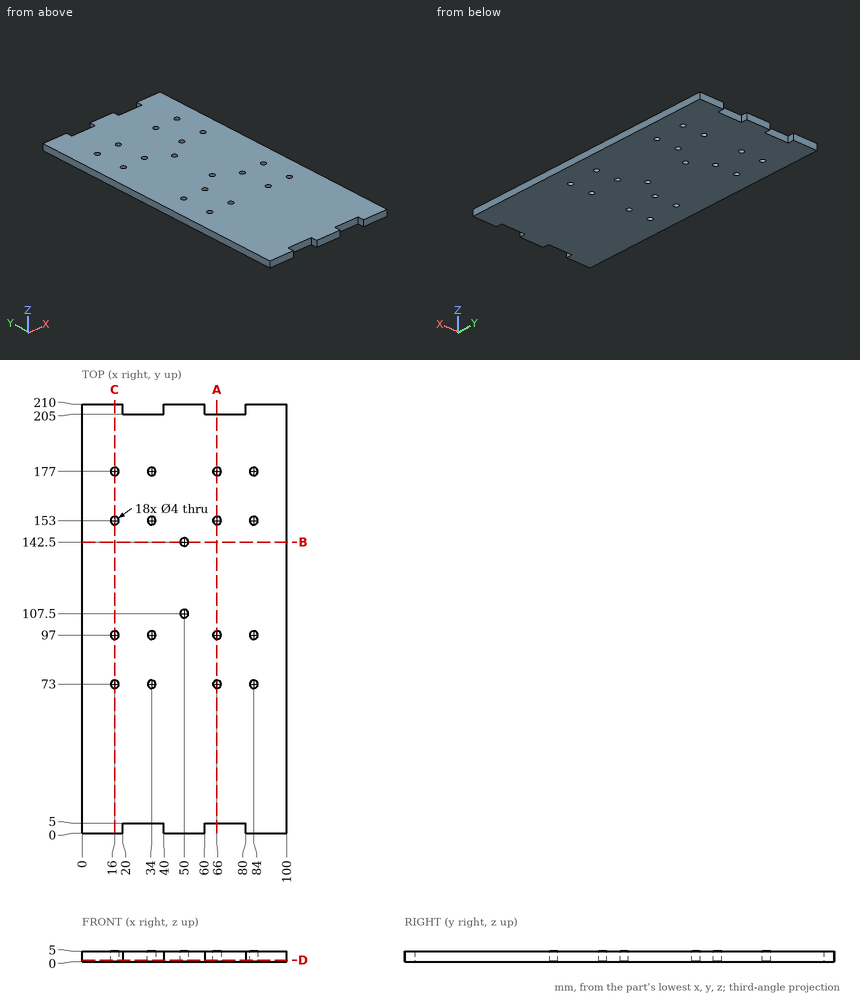
Verification items for this drawing (mm, ordinates from the low corner). Coordinates: 2 decimals unless noted, no trailing zeros. Write each loop counter-clockwise with the first axis right and the second up, starting at its lowest first coordinate (ties: lowest second). Pieces come first, ordered by that corner, then holes. Notation, with made-up numbers: M 63,18.5 L 70,18.5 A26 ccw 70,39.5 Z; hole C 81.5,10 d8. An arc over 180 degrees is marked long. Answer as CSV lines item,"result".
Q1. Cross-section at C-C (x = 16). Record the boundary of the cut face in (y, z).
Check result:
outline,"M 0,0 L 71,0 L 71,5 L 0,5 Z; M 75,0 L 95,0 L 95,5 L 75,5 Z; M 99,0 L 151,0 L 151,5 L 99,5 Z; M 155,0 L 175,0 L 175,5 L 155,5 Z; M 179,0 L 210,0 L 210,5 L 179,5 Z"
Q2. Cross-section at A-A (x = 66). Record the boundary of the cut face in (y, z).
Check result:
outline,"M 5,0 L 71,0 L 71,5 L 5,5 Z; M 75,0 L 95,0 L 95,5 L 75,5 Z; M 99,0 L 151,0 L 151,5 L 99,5 Z; M 155,0 L 175,0 L 175,5 L 155,5 Z; M 179,0 L 205,0 L 205,5 L 179,5 Z"
Q3. Material ranges on probe 1 along Y at (x, z) = (16, 1.85); probe 2 along Y at (x, z) = (66, 1.3); probe 3 along X at (y, z) = (153, 3.35), recorded low to high. Write a range as from..to.
Check result:
probe 1,"0..71, 75..95, 99..151, 155..175, 179..210"
probe 2,"5..71, 75..95, 99..151, 155..175, 179..205"
probe 3,"0..14, 18..32, 36..64, 68..82, 86..100"
Q4. Cross-section at B-B (y = 142.5). Record the boundary of the cut face in (x, z).
Check result:
outline,"M 0,0 L 48,0 L 48,5 L 0,5 Z; M 52,0 L 100,0 L 100,5 L 52,5 Z"
Q5. Cross-section at D-D (z = 0.75). Count the separate pieces of the cut face and the enclosed holes in it, then the cut area to 3 significant figures.
Check result:
separate pieces,"1"
enclosed holes,"18"
area,"20,400 mm^2"
Q6. Go/stop test with a flat-tipped pin: pin 1 (1 mm diameter, centred on x = 26.5, z = 4, fed in from -Y). Record where the tip stops, or that it passes through.
Check result:
pin 1,"y = 5"
